The figure shows three views and two pictorial views of one solid part (mm, origin at its lowest corner). Answer the questions. A direction names the side the tool comes from. Coordinates: 2 decimals unless noted, no trailing zeros. Write each loop counter-clockwise with the first axis right and the second up, starting at its lowest first coordinate (ties: lowest second). Pieces come first, ordered by that corner, then holes.
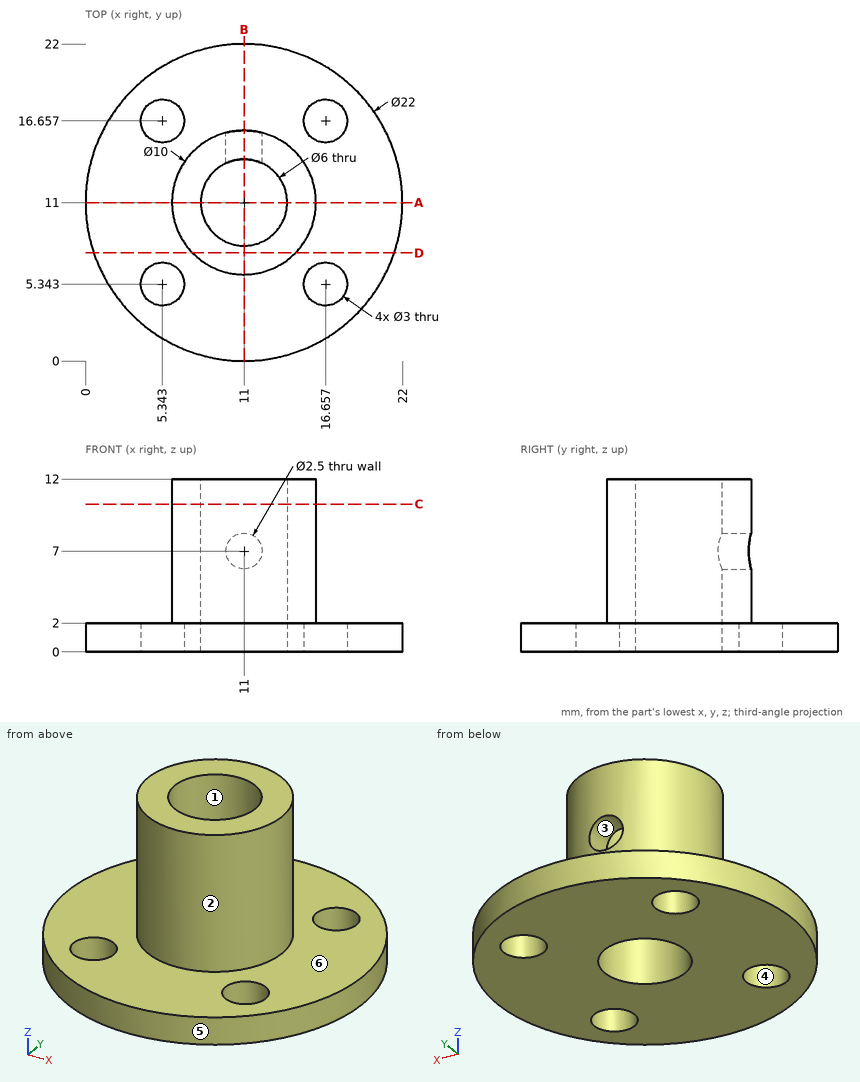
Q1. The part is cut by section C-C, the plane z = 10.25. Write down the section's boundary in (x, y).
Answers below:
outline: circle Ø10 at (11, 11); hole circle Ø6 at (11, 11)
Q2. Determine the mould class of the marked faces 3, 4, 5 and 6 for opening direction X: released by +X, released by -X, zero draft, split by the parting line, or undercut.
Answers below:
face 3: undercut
face 4: undercut
face 5: split by the parting line
face 6: zero draft
Q3. The part is cut by section B-B, the plane x = 11. Write down the section's boundary in (y, z), then the cut area to 3 significant figures.
Answers below:
outline: (0, 0) - (8, 0) - (8, 12) - (6, 12) - (6, 2) - (0, 2) - close; (14, 0) - (22, 0) - (22, 2) - (16, 2) - (16, 5.75) - (14, 5.75) - close; (14, 8.25) - (16, 8.25) - (16, 12) - (14, 12) - close
area: 67.0 mm2
Q4. The part is cut by section A-A, the plane y = 11. Write down the section's boundary in (x, z), then the cut area to 3 significant figures.
Answers below:
outline: (0, 0) - (8, 0) - (8, 12) - (6, 12) - (6, 2) - (0, 2) - close; (14, 0) - (22, 0) - (22, 2) - (16, 2) - (16, 12) - (14, 12) - close
area: 72.0 mm2
Q5. The part is cut by section D-D, the plane y = 7.5. Write down the section's boundary in (x, z).
Answers below:
outline: (0.57, 0) - (21.43, 0) - (21.43, 2) - (14.57, 2) - (14.57, 12) - (7.43, 12) - (7.43, 2) - (0.57, 2) - close
Q6. Find the intervals of material crossed by probe 1 along Y at (x, z) = (4.5, 0.5); probe 2 along X at (y, z) = (13, 8.25); probe 3 along Y at (x, z) = (12.25, 9), in increasing order.
Answers below:
probe 1: y = 2.13 to 4.1, 6.58 to 15.42, 17.9 to 19.87
probe 2: x = 6.42 to 8.76, 13.24 to 15.58
probe 3: y = 6.16 to 8.27, 13.73 to 15.84
Q7. Given pin 1 (6 mm diameter, centred on x = 6.5, z = 6.5, fed in from +Y); pin 2 (11 mm diameter, centred on x = 6, y = 15.5, fed in from +Z); pin 3 (4 mm diameter, centred on x = 5.34, y = 16.66, fed in from +Z); pin 4 (1.5 mm diameter, centred on x = 16, z = 5.5, fed in from +Y), each flat-ended and moving along its own axis, determine where each tip first touches the part or whether it passes through.
Answers below:
pin 1: stops at y = 15.77
pin 2: stops at z = 12
pin 3: stops at z = 2
pin 4: stops at y = 13.63
Q8. Which of the six approach directions +Z, -Z, +X, -X, +Y, -Y give full straight-line access (tool end or side, diameter ignored) to the marked faces 1 and 2?
Answers below:
face 1: +Z, -Z
face 2: +Z
